Can you work these out from the model? Positions are in its coordinate system, mm. A direction names the side the tool comes from. Coordinates: 2 decimals unless noted, no trailing zeros. Loops run counter-clockwise (first coordinate to the right, second up) from the corner with the lowest first, then second, coordinate; pieces in that order, holes last.
```python
from build123d import *

# Parameters (mm, degrees)
CUT_EXTRUDE1_DEPTH       = 5
CUT_EXTRUDE3_DEPTH       = 45
SKETCH8_R                = 40
CUT_EXTRUDE4_DEPTH       = 32
SKETCH9_R                = 32
SKETCH9_R_2              = 24.5
CUT_EXTRUDE5_DEPTH       = 14
SKETCH10_R               = 26
CUT_EXTRUDE6_DEPTH       = 14
FILLET1_R                = 7
FILLET2_R                = 7
CUT_REVOLVE1_START       = 22
CUT_REVOLVE1_DEPTH       = 30.5
CUT_EXTRUDE12_DEPTH      = 5
SKETCH18_W               = 13
SKETCH18_H               = 8
CUT_EXTRUDE13_DEPTH      = 5
INTERSECT1_OUTLINE_R     = 42
INTERSECT1_DEPTH         = 55
SKETCH20_W               = 6
SKETCH20_H               = 3
BOSS_EXTRUDE1_DEPTH      = 8
BOSS_EXTRUDE2_DEPTH      = 1
BOSS_EXTRUDE2_DEPTH_BACK = 1
SKETCH21_W               = 6
SKETCH21_H               = 6
BOSS_EXTRUDE3_DEPTH      = 7
SKETCH19_R               = 1.5
CUT_EXTRUDE14_DEPTH      = 20
SKETCH23_W               = 20
SKETCH23_H               = 7
CUT_EXTRUDE15_DEPTH      = 7
SKETCH24_W               = 44
SKETCH24_H               = 3.5
CUT_EXTRUDE16_DEPTH      = 5
FILLET3_R                = 2


# Read off the part's stored shape, not the designer's step: Cut-Revolve1, Intersect1
with BuildPart() as part:
    # Sketch1 → Revolve1 (revolve)
    with BuildSketch(Plane.XY, mode=Mode.PRIVATE) as revolve1_sk:
        with BuildLine():
            Line((22.5, 0), (32, 0))
            ThreePointArc((32, 0), (33.414213562, 0.585786438), (34, 2))
            Line((34, 2), (34, 18))
            Line((34, 18), (40, 18))
            ThreePointArc((40, 18), (41.414213562, 18.585786438), (42, 20))
            Line((42, 20), (42, 55))
            ThreePointArc((42, 55), (40.535533906, 58.535533906), (37, 60))
            Line((37, 60), (0, 60))
            Line((0, 60), (0, 18))
            Line((0, 18), (22.5, 18))
            Line((22.5, 18), (22.5, 0))
        make_face()
    revolve(revolve1_sk.sketch.rotate(Axis((0, 2, 0), (0, 1, 0)), 90), axis=Axis((0, 2, 0), (0, 1, 0)))

    # Sketch5 → Cut-Extrude1 (cut)
    with BuildSketch(Plane(origin=(0, 60, 0), x_dir=(1, 0, 0), z_dir=(0, 1, 0))):
        with BuildLine():
            Line((-42, 0), (-40, 0))
            Line((-40, 0), (40, 0))
            Line((40, 0), (42, 0))
            ThreePointArc((42, 0), (0, 42), (-42, 0))
        make_face()
    extrude(amount=-CUT_EXTRUDE1_DEPTH, mode=Mode.SUBTRACT)

    # Sketch7 → Cut-Extrude3 (cut)
    with BuildSketch(Plane.XZ.offset(-18)):
        with BuildLine():
            Line((-21, 0), (21, 0))
            ThreePointArc((21, 0), (0, -21), (-21, 0))
        make_face()
    extrude(amount=-CUT_EXTRUDE3_DEPTH, mode=Mode.SUBTRACT)

    # Sketch8 → Cut-Extrude4 (cut)
    with BuildSketch(Plane(origin=(0, 52.5, 0), x_dir=(1, 0, 0), z_dir=(0, 1, 0))):
        with Locations(Location((0, 0, 0), (0, 0, 270))):
            Circle(SKETCH8_R)
        with BuildLine():
            Line((22.912878475, -2), (-22.912878475, -2))
            ThreePointArc((-22.912878475, -2), (0, 23), (22.912878475, -2))
        make_face(mode=Mode.SUBTRACT)
    extrude(amount=-CUT_EXTRUDE4_DEPTH, mode=Mode.SUBTRACT)

    # Sketch9 → Cut-Extrude5 (cut)
    with BuildSketch(Plane(origin=(0, 2, 0), x_dir=(-1, 0, 0), z_dir=(0, -1, 0))):
        with Locations(Location((0, 0, 0), (0, 0, 90))):
            Circle(SKETCH9_R)
        with Locations(Location((0, 0, 0), (0, 0, 90))):
            Circle(SKETCH9_R_2, mode=Mode.SUBTRACT)
    extrude(amount=-CUT_EXTRUDE5_DEPTH, mode=Mode.SUBTRACT)

    # Sketch10 → Cut-Extrude6 (cut)
    with BuildSketch(Plane(origin=(0, 2, 0), x_dir=(-1, 0, 0), z_dir=(0, -1, 0))):
        Circle(SKETCH10_R)
    extrude(amount=-CUT_EXTRUDE6_DEPTH, mode=Mode.SUBTRACT)

    # Fillet1
    fillet1_edges = [part.edges().sort_by_distance(p)[0] for p in [
        (21, 36.5, 0),
        (-21, 36.5, 0),
    ]]
    fillet(fillet1_edges, radius=FILLET1_R)

    # Fillet2
    fillet2_edges = [part.edges().sort_by_distance(p)[0] for p in [
        (-22.912878475, 36.5, 2),
        (22.912878475, 36.5, 2),
    ]]
    fillet(fillet2_edges, radius=FILLET2_R)

    # Cut-Revolve1 outline → Cut-Revolve1 (cut)
    with BuildSketch(Plane(origin=(0, 0, 0), x_dir=(1, 0, 0), z_dir=(0, 1, 0)).offset(CUT_REVOLVE1_START)):
        with BuildLine():
            Line((-34.641016151, -20), (-36.373066959, -21))
            ThreePointArc((-36.373066959, -21), (0, -42), (36.373066959, -21))
            Line((36.373066959, -21), (34.641016151, -20))
            ThreePointArc((34.641016151, -20), (0, -40), (-34.641016151, -20))
        make_face()
    extrude(amount=CUT_REVOLVE1_DEPTH, mode=Mode.SUBTRACT)

    # Sketch15 → Cut-Extrude12 (cut)
    with BuildSketch(Plane(origin=(0, 20.5, 0), x_dir=(1, 0, 0), z_dir=(0, 1, 0))):
        with BuildLine():
            Line((-28.124355653, -3.514579578), (-26.124355653, -3.514579578))
            ThreePointArc((-26.124355653, -3.514579578), (-24.710142091, -2.928793141), (-24.124355653, -1.514579578))
            Line((-24.124355653, -1.514579578), (-24.124355653, 8.485420422))
            ThreePointArc((-24.124355653, 8.485420422), (-24.710142091, 9.899633984), (-26.124355653, 10.485420422))
            Line((-26.124355653, 10.485420422), (-28.124355653, 10.485420422))
            ThreePointArc((-28.124355653, 10.485420422), (-29.538569215, 9.899633984), (-30.124355653, 8.485420422))
            Line((-30.124355653, 8.485420422), (-30.124355653, -1.514579578))
            ThreePointArc((-30.124355653, -1.514579578), (-29.538569215, -2.928793141), (-28.124355653, -3.514579578))
        make_face()
    extrude(amount=-CUT_EXTRUDE12_DEPTH, mode=Mode.SUBTRACT)

    # Sketch18 → Cut-Extrude13 (cut)
    with BuildSketch(Plane(origin=(0, 55, 0), x_dir=(1, 0, 0), z_dir=(0, 1, 0))):
        with Locations((0.796512215, 32.951769165)):
            Rectangle(SKETCH18_W, SKETCH18_H)
    extrude(amount=-CUT_EXTRUDE13_DEPTH, mode=Mode.SUBTRACT)

    # Intersect1 outline → Intersect1 (cut)
    with BuildSketch(Plane(origin=(0, 0, 0), x_dir=(1, 0, 0), z_dir=(0, 1, 0))):
        Circle(INTERSECT1_OUTLINE_R)
        with BuildLine():
            Line((12.124355653, 0), (-12.124355653, 0))
            ThreePointArc((-12.124355653, 0), (-18.186533479, 3.5), (-18.186533479, 10.5))
            ThreePointArc((-18.186533479, 10.5), (0, 21), (18.186533479, 10.5))
            ThreePointArc((18.186533479, 10.5), (18.186533479, 3.5), (12.124355653, 0))
        make_face(mode=Mode.SUBTRACT)
    extrude(amount=INTERSECT1_DEPTH, mode=Mode.SUBTRACT)

    # Sketch20 → Boss-Extrude1 (add)
    with BuildSketch(Plane.XZ.offset(-55)):
        with Locations((0, 33.5)):
            Rectangle(SKETCH20_W, SKETCH20_H)
    extrude(amount=BOSS_EXTRUDE1_DEPTH)

    # Sketch21 → Boss-Extrude2 (add, two sides: drawn at the far end of the back side and taken through both)
    with BuildSketch(Plane.XZ.offset(-47).offset(-BOSS_EXTRUDE2_DEPTH_BACK)):
        with Locations((0, 32)):
            Rectangle(SKETCH21_W, SKETCH21_H)
    extrude(amount=BOSS_EXTRUDE2_DEPTH + BOSS_EXTRUDE2_DEPTH_BACK)

    # Sketch22 → Boss-Extrude3 (add)
    with BuildSketch(Plane(origin=(0, 0, 0), x_dir=(-1, 0, 0), z_dir=(0, 0, -1))):
        with BuildLine():
            Line((-42, 55), (42, 55))
            ThreePointArc((42, 55), (40.535533906, 58.535533906), (37, 60))
            Line((37, 60), (-37, 60))
            ThreePointArc((-37, 60), (-40.535533906, 58.535533906), (-42, 55))
        make_face()
    extrude(amount=BOSS_EXTRUDE3_DEPTH)

    # Sketch19 → Cut-Extrude14 (cut)
    with BuildSketch(Plane(origin=(0, 0, -7), x_dir=(-1, 0, 0), z_dir=(0, 0, -1))):
        with Locations((0, 57.5)):
            Circle(SKETCH19_R)
        with Locations((-30, 57.5)):
            Circle(SKETCH19_R)
        with Locations((30, 57.5)):
            Circle(SKETCH19_R)
    extrude(amount=-CUT_EXTRUDE14_DEPTH, mode=Mode.SUBTRACT)

    # Sketch23 → Cut-Extrude15 (cut)
    with BuildSketch(Plane(origin=(0, 60, 0), x_dir=(1, 0, 0), z_dir=(0, 1, 0))):
        with Locations((-32, 3.5)):
            Rectangle(SKETCH23_W, SKETCH23_H)
        with Locations((32, 3.5)):
            Rectangle(SKETCH23_W, SKETCH23_H)
    extrude(amount=-CUT_EXTRUDE15_DEPTH, mode=Mode.SUBTRACT)

    # Sketch24 → Cut-Extrude16 (cut)
    with BuildSketch(Plane(origin=(0, 60, 0), x_dir=(1, 0, 0), z_dir=(0, 1, 0))):
        with Locations((0, 5.25)):
            Rectangle(SKETCH24_W, SKETCH24_H)
    extrude(amount=-CUT_EXTRUDE16_DEPTH, mode=Mode.SUBTRACT)

    # Fillet3
    # the kernel refuses this fillet: 2 mm, written as the material it takes off along each edge
    with BuildSketch(Plane(origin=(27, 55, -3.5), x_dir=(0, 0, 1), z_dir=(-1, 0, 0))) as fillet3_piece_1:
        with BuildLine():
            CenterArc((FILLET3_R, FILLET3_R), FILLET3_R, 180, 90)
            Line((0, FILLET3_R), (0, 0))
            Line((0, 0), (FILLET3_R, 0))
        make_face()
    extrude(amount=54, mode=Mode.SUBTRACT)


solid = part.part
```
Item 1: I need wall thicknesses on line 1 along Y through (x, z) = (-30, 9.75); line 2 along Y through (x, z) = (-8.5, 30); line 3 along X through (y, z) = (58, -2). Which ranges of each line are inside material? Lowest first, please.
Results are:
line 1: y = 55 to 56, 59 to 60
line 2: y = 55 to 60
line 3: x = -22 to -1.41, 1.41 to 22
Item 2: I'm going to push flat-ended pins straight in: P1, Ø1.5, axis at x = -34, y = 58, coming from the -Z side; P2, Ø3, axis at x = -26, z = 28, coming from the -Y side; P3, Ø1.5, axis at x = 30.5, y = 58, coming from the -Z side. Where does each tip first touch, or does it pass through?
Results are:
P1: stops at z = 0
P2: stops at y = 55
P3: stops at z = 13
Item 3: Suppose I cut it at A-A, the plane x = 0. Please give me the cut outline in (y, z), plus the area to 3 significant figures.
Results are:
outline: (46, 29) - (48, 29) - (48, 32) - (55, 32) - (55, -1.5) arc R2 ccw to (56, -3.23) - (56, 13) - (59, 13) - (59, -3.5) - (60, -3.5) - (60, 37) arc R5 ccw to (55, 42) - (55, 35) - (46, 35) - close
area: 205 mm2
Item 4: On a 3-axis mill with a long thin cutter (end or side, diameter ignored), from which of +Z, -Z, +X, -X, +Y, -Y can I reach the whole of each face in a straight line? I mean faces 5 (the face through (-22, 58, -2)), 6 (the face through (0, 58, 13)), 7 (the face through (0, 52, 32)), 8 (the face through (0, 51, 35)), 9 (the face through (32, 58, 0)). Say none if no direction works.
Results are:
face 5: -Z, -X, +Y, -Y
face 6: -Z
face 7: -Z, +X, -X
face 8: +Z, +X, -X, -Y
face 9: -Z, +X, +Y, -Y
Item 5: We'd pull the mould along X, two halves only. Please class faces 1 (the face through (30, 58, 13)), 2 (the face through (3, 50, 33)), 3 (the face through (-30, 58, 13)), 4 (the face through (0, 47, 29)): +X half, -X half, draft (parallel to the pull), parting line (faces both ways), or undercut.
Results are:
face 1: undercut
face 2: +X half
face 3: undercut
face 4: draft
Item 6: Suppose I cut it at C-C, the plane y = 53. Please give me the cut outline in (x, z).
Results are:
outline: (-3, 32) - (3, 32) - (3, 35) - (-3, 35) - close
Item 7: Suppose I cut it at B-B, the plane z = 12. Count the separate pieces of the cut face and the enclosed holes in it, plus the area to 3 significant figures.
Results are:
separate pieces: 1
enclosed holes: 3
area: 370 mm2
